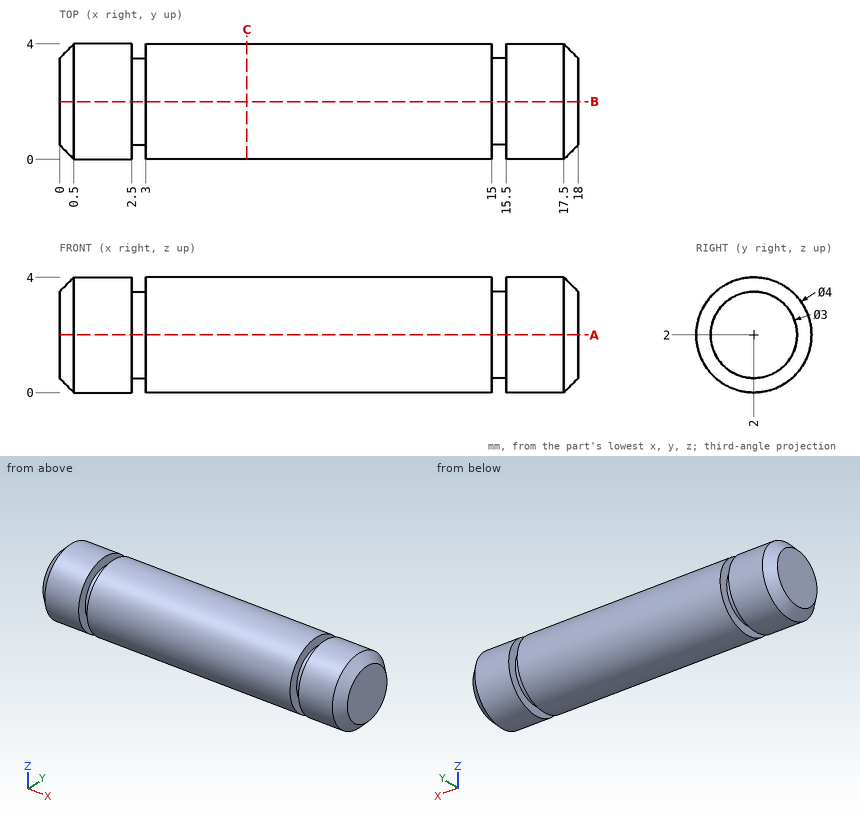
Check sheet for the drawn part. Datum: minimum x, y, z corner. Units: mm. Round coordinates to 2 decimals unless told otherwise and drop trailing zeros. Loops run counter-clockwise (first coordinate to the right, second up) from the corner with the lowest first, then second, coordinate; pieces in that order, holes last.
Item 1: Thickness scan on line 1 (Z direction, x = 1.5, y = 0.3); line 2 (Z direction, x = 2.25, y = 2.95); line 3 (Y direction, x = 6.5, z = 1.55). Record the ranges inside material, lowest first.
Item 2: Gauge pin test, flat end, axial feed: pin 1 (2 mm diameter, centred on y = 1.5, z = 3, fed in from -X). Record the tip position at first contact, or that the pin passes through.
Item 3: Cross-section at C-C on x = 6.5. Record the boundary of the cut face in (y, z), then the cut area to 3 significant figures.
Item 4: Cross-section at A-A on z = 2. Record the boundary of the cut face in (x, y), then the cut area to 3 significant figures.
Answer sheet:
1. line 1: z = 0.95 to 3.05
1. line 2: z = 0.24 to 3.76
1. line 3: y = 0.05 to 3.95
2. pin 1: stops at x = 0
3. outline: circle Ø4 at (2, 2)
3. area: 12.6 mm2
4. outline: (0, 0.5) - (0.5, 0) - (2.5, 0) - (2.5, 0.5) - (3, 0.5) - (3, 0) - (15, 0) - (15, 0.5) - (15.5, 0.5) - (15.5, 0) - (17.5, 0) - (18, 0.5) - (18, 3.5) - (17.5, 4) - (15.5, 4) - (15.5, 3.5) - (15, 3.5) - (15, 4) - (3, 4) - (3, 3.5) - (2.5, 3.5) - (2.5, 4) - (0.5, 4) - (0, 3.5) - close
4. area: 70.5 mm2
